Work out the finished part from the listing and answer in its coordinate system (mm). Face numbers are marked on the shaded views. A direction names the side the tool comes from. Coordinates: 2 decimals unless noted, no trailing zeros. Loops run counter-clockwise (first coordinate to the right, second up) from the corner with the lowest first, then second, coordinate; pieces in that order, holes last. Notation, with made-up numbers: (-11, 36) -> (40, 36) arc R26 ccw to (40, 63) -> close; hole circle Ø3 at (62, -22). An arc over 180 degrees is marked (long way). Use a Markdown table: item, result.
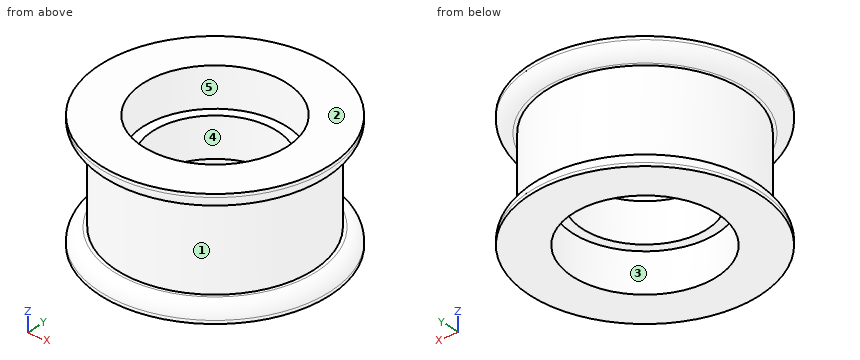
from build123d import *

# Parameters (mm, degrees)
SKETCH_1_R          = 15
EXTRUDE_1_DEPTH     = 6.5
SKETCH_2_R          = 17.5
EXTRUDE_2_DEPTH     = 2.5
SKETCH_3_R          = 11
CUT_EXTRUDE_1_DEPTH = 6
CUT_EXTRUDE_START   = -6
SKETCH_4_R          = 11
CUT_EXTRUDE_2_DEPTH = 6
SKETCH_5_R          = 9.5
CUT_EXTRUDE_3_DEPTH = 28.504545079
FILLET_1_R          = 2


with BuildPart() as part:
    # 草图1 → 拉伸1 (new, symmetric)
    with BuildSketch(Plane.XY):
        with Locations(Location((0, 0, 0), (0, 0, 180))):
            Circle(SKETCH_1_R)
    extrude(amount=EXTRUDE_1_DEPTH, both=True)

    # 草图2 → 拉伸2 (add)
    with BuildSketch(Plane.XY.offset(6.5)):
        Circle(SKETCH_2_R)
    extrude_2 = extrude(amount=EXTRUDE_2_DEPTH)

    # 镜向1: 拉伸2 across plane
    add(extrude_2.mirror(Plane.XY))

    # 草图3 → 切除-拉伸1 (cut)
    with BuildSketch(Plane.XY.offset(9)):
        Circle(SKETCH_3_R)
    extrude(amount=-CUT_EXTRUDE_1_DEPTH, mode=Mode.SUBTRACT)

    # 草图4 → 切除-拉伸2 (cut)
    with BuildSketch(Plane(origin=(0, 0, -9), x_dir=(-1, 0, 0), z_dir=(0, 0, -1)).offset(CUT_EXTRUDE_START)):
        with Locations(Location((0, 0, 0), (0, 0, 180))):
            Circle(SKETCH_4_R)
    extrude(amount=CUT_EXTRUDE_2_DEPTH, mode=Mode.SUBTRACT)

    # 草图5 → 切除-拉伸3 (cut, through all)
    with BuildSketch(Plane(origin=(0, 0, -3), x_dir=(-1, 0, 0), z_dir=(0, 0, -1))):
        Circle(SKETCH_5_R)
    extrude(amount=-CUT_EXTRUDE_3_DEPTH, mode=Mode.SUBTRACT)

    # 圆角1
    fillet_1_edges = [part.edges().sort_by_distance(p)[0] for p in [
        (-17.5, 0, 6.5),
        (-17.5, 0, -6.5),
    ]]
    fillet(fillet_1_edges, radius=FILLET_1_R)


solid = part.part
Q1. Given pin 1 Ø1.5 at (x, y) = (4, -6) entering from +Z; pin 2 Ø6 at (x, y) = (3.5, -7) entering from +Z; pin 3 Ø3 at (y, z) = (11, -4) entering from -X; pin 4 Ø5 at (x, z) = (-2, 5.5) entering from +Y, each flat-ended and moving along its own axis, determine where each tip first touches the part or whether it passes through.
Solved:
| item | result |
|---|---|
| pin 1 | through |
| pin 2 | z = 3 |
| pin 3 | x = -11.61 |
| pin 4 | y = 17.36 |
Q2. Determine the mould class of the marked faces 1, 2 and 3 for opening direction X: pulls with the +X half, pulls with the -X half, needs draft (parallel to the pull), parting line crosses it, or undercut.
Solved:
| item | result |
|---|---|
| face 1 | parting line crosses it |
| face 2 | needs draft |
| face 3 | undercut |
Q3. Section C-C on z = -5.5 is taken. Determine the outline of the cut face in (x, y), and give its area (3 significant figures).
Solved:
| item | result |
|---|---|
| outline | circle Ø30 at (0, 0); hole circle Ø22 at (0, 0) |
| area | 327 mm² |
Q4. For the marked faces 4 and 5, determine the directions among +Z, -Z, +X, -X, +Y, -Y from which every point of the face is accessible in a straight line to the end or side of a thin tool.
Solved:
| item | result |
|---|---|
| face 4 | +Z, -Z |
| face 5 | +Z |
Q5. Section A-A on y = 0 is taken. Determine the outline of the cut face in (x, z), and give its area (3 significant figures).
Solved:
| item | result |
|---|---|
| outline | (-17.5, -9) -> (-11, -9) -> (-11, -3) -> (-9.5, -3) -> (-9.5, 3) -> (-11, 3) -> (-11, 9) -> (-17.5, 9) -> (-17.5, 8.5) arc R2 ccw to (-15.5, 6.5) -> (-15, 6.5) -> (-15, -6.5) -> (-15.5, -6.5) arc R2 ccw to (-17.5, -8.5) -> close; (9.5, -3) -> (11, -3) -> (11, -9) -> (17.5, -9) -> (17.5, -8.5) arc R2 ccw to (15.5, -6.5) -> (15, -6.5) -> (15, 6.5) -> (15.5, 6.5) arc R2 ccw to (17.5, 8.5) -> (17.5, 9) -> (11, 9) -> (11, 3) -> (9.5, 3) -> close |
| area | 184 mm² |
Q6. Consider line 1 (Y direction, x = 0, z = -4.4); line 2 (Y direction, x = 0, z = 0.85); line 3 (X direction, y = -6.5, z = -1). Determine where each line is inside the solid, lowest interval first. Write a range as [from, to].
Solved:
| item | result |
|---|---|
| line 1 | [-15, -11], [11, 15] |
| line 2 | [-15, -9.5], [9.5, 15] |
| line 3 | [-13.52, -6.93], [6.93, 13.52] |
Q7. Section D-D on z = 2.25 is taken. Determine the outline of the cut face in (x, y).
Solved:
| item | result |
|---|---|
| outline | circle Ø30 at (0, 0); hole circle Ø19 at (0, 0) |
